from build123d import *

# Parameters (mm, degrees)
BRIDA_BASE1_DEPTH                = 2
REDONDEO5MM_R                    = 5
REDONDEO3MM_R                    = 3
BRIDA_DE_ARISTA1_STRIP_W         = 12
BRIDA_DE_ARISTA1_STRIP_H         = 2
BRIDA_DE_ARISTA1_STRIP_CUT_DEPTH = 30
BRIDA_DE_ARISTA1_DEPTH           = 30
BRIDA_DE_ARISTA2_STRIP_W         = 12
BRIDA_DE_ARISTA2_STRIP_H         = 2
BRIDA_DE_ARISTA2_STRIP_CUT_DEPTH = 18
BRIDA_DE_ARISTA2_DEPTH           = 18
BRIDA_START                      = 2
BRIDA_DE_ARISTA2_FLAT_DEPTH      = 2
CORTAR_EXTRUIR6_REACH            = 43.255
CROQUIS26_R                      = 2
REDONDEO11MM_R                   = 11
TALADRO_ROSCADO_M32_D            = 2.5
TALADRO_ROSCADO_M32_DEPTH        = 20.65
TALADRO_ROSCADO_M32_TIP          = 0.751075774
TALADRO_ROSCADO_M52_D            = 4.2
TALADRO_ROSCADO_M52_DEPTH        = 2
CORTAR_EXTRUIR7_REACH            = 42.274
CROQUIS36_R                      = 2


# Sheet-metal steps are written as plain solids
with BuildPart() as part:
    # Croquis1 → Brida base1 (new body)
    with BuildSketch(Plane.XY):
        with BuildLine():
            Line((0, 0), (30, 0))
            Line((30, 0), (30, 3))
            ThreePointArc((30, 3), (27.886584846, 9.212566007), (24, 14.5))
            Line((24, 14.5), (24, 17))
            Line((24, 17), (6, 17))
            Line((6, 17), (6, 14.5))
            ThreePointArc((6, 14.5), (2.113415154, 9.212566007), (0, 3))
            Line((0, 3), (0, 0))
        make_face()
    extrude(amount=-BRIDA_BASE1_DEPTH)

    # Redondeo5mm
    redondeo5mm_edges = [part.edges().sort_by_distance(p)[0] for p in [
        (0, 3, -1),
        (30, 3, -1),
    ]]
    fillet(redondeo5mm_edges, radius=REDONDEO5MM_R)

    # Redondeo3mm
    redondeo3mm_edges = [part.edges().sort_by_distance(p)[0] for p in [
        (6, 14.5, -1),
        (24, 14.5, -1),
    ]]
    fillet(redondeo3mm_edges, radius=REDONDEO3MM_R)

    # Brida de arista1 strip (across the edge) → Brida de arista1 strip cut (cut)
    with BuildSketch(Plane.YZ):
        with Locations((-4, -1)):
            Rectangle(BRIDA_DE_ARISTA1_STRIP_W, BRIDA_DE_ARISTA1_STRIP_H)
    extrude(amount=BRIDA_DE_ARISTA1_STRIP_CUT_DEPTH, mode=Mode.SUBTRACT)

    # Brida de arista1 section (across the edge) → Brida de arista1 (add)
    with BuildSketch(Plane.YZ):
        with BuildLine():
            Line((-2, 2), (-2, 19))
            Line((-2, 19), (0, 19))
            Line((0, 19), (0, 2))
            ThreePointArc((0, 2), (0.585786438, 0.585786438), (2, 0))
            Line((2, 0), (2, -2))
            ThreePointArc((2, -2), (-0.828427125, -0.828427125), (-2, 2))
        make_face()
    extrude(amount=BRIDA_DE_ARISTA1_DEPTH)

    # Brida de arista2 strip (across the edge) → Brida de arista2 strip cut (cut)
    with BuildSketch(Plane(origin=(24, 17, 0), x_dir=(0, -1, 0), z_dir=(-1, 0, 0))):
        with Locations((-4, -1)):
            Rectangle(BRIDA_DE_ARISTA2_STRIP_W, BRIDA_DE_ARISTA2_STRIP_H)
    extrude(amount=BRIDA_DE_ARISTA2_STRIP_CUT_DEPTH, mode=Mode.SUBTRACT)

    # Brida de arista2 bend section (across the edge) → Brida de arista2 (add)
    with BuildSketch(Plane(origin=(24, 17, 0), x_dir=(0, -1, 0), z_dir=(-1, 0, 0))):
        with BuildLine():
            Line((-2, 2), (0, 2))
            ThreePointArc((0, 2), (0.585786438, 0.585786438), (2, 0))
            Line((2, 0), (2, -2))
            ThreePointArc((2, -2), (-0.828427125, -0.828427125), (-2, 2))
        make_face()
    extrude(amount=BRIDA_DE_ARISTA2_DEPTH)

    # Brida de arista2 profile (on flange) → Brida de arista2 flat (add)
    with BuildSketch(Plane(origin=(0, 17, 0), x_dir=(-1, 0, 0), z_dir=(0, 1, 0)).offset(BRIDA_START)):
        with BuildLine():
            ThreePointArc((-6, 10), (-15, 19), (-24, 10))
            Line((-24, 10), (-24, 2))
            Line((-24, 2), (-6, 2))
            Line((-6, 2), (-6, 10))
        make_face()
    extrude(amount=-BRIDA_DE_ARISTA2_FLAT_DEPTH)

    # Croquis26 → Cortar-Extruir6 (cut, up to next)
    with BuildSketch(Plane(origin=(0, 0, -2), x_dir=(-1, 0, 0), z_dir=(0, 0, -1)), mode=Mode.PRIVATE) as cortar_extruir6_sk1:
        with Locations((-6.25, 8.3)):
            Circle(CROQUIS26_R)
    cortar_extruir6_tool1 = extrude(cortar_extruir6_sk1.sketch, amount=-CORTAR_EXTRUIR6_REACH, mode=Mode.PRIVATE) & part.part
    # Croquis26 → Cortar-Extruir6 (cut, up to next)
    with BuildSketch(Plane(origin=(0, 0, -2), x_dir=(-1, 0, 0), z_dir=(0, 0, -1)), mode=Mode.PRIVATE) as cortar_extruir6_sk2:
        with Locations((-23.75, 8.3)):
            Circle(CROQUIS26_R)
    cortar_extruir6_tool2 = extrude(cortar_extruir6_sk2.sketch, amount=-CORTAR_EXTRUIR6_REACH, mode=Mode.PRIVATE) & part.part
    add(cortar_extruir6_tool1.solids().sort_by_distance((6.25, 8.3, -2))[0], mode=Mode.SUBTRACT)
    add(cortar_extruir6_tool2.solids().sort_by_distance((23.75, 8.3, -2))[0], mode=Mode.SUBTRACT)

    # Redondeo11mm
    redondeo11mm_edges = [part.edges().sort_by_distance(p)[0] for p in [
        (0, -1, 19),
        (30, -1, 19),
    ]]
    fillet(redondeo11mm_edges, radius=REDONDEO11MM_R)

    # Taladro roscado M32
    with Locations(Plane(origin=(0, 0, 0), x_dir=(1, 0, 0), z_dir=(0, 1, 0))):
        with Locations((3.25, -9), (26.75, -9)):
            Hole(TALADRO_ROSCADO_M32_D / 2, depth=TALADRO_ROSCADO_M32_DEPTH)
            with Locations((0, 0, -(TALADRO_ROSCADO_M32_DEPTH + TALADRO_ROSCADO_M32_TIP / 2))):  # 118° drill point
                Cone(0, TALADRO_ROSCADO_M32_D / 2, TALADRO_ROSCADO_M32_TIP, mode=Mode.SUBTRACT)

    # Taladro roscado M52
    with Locations(Plane(origin=(3.715500562, 0, 2.638137214), x_dir=(1, 0, 0), z_dir=(0, 1, 0))):
        with Locations((11.284499438, -7.361862786)):
            Hole(TALADRO_ROSCADO_M52_D / 2, depth=TALADRO_ROSCADO_M52_DEPTH)

    # Croquis36 → Cortar-Extruir7 (cut, up to next)
    with BuildSketch(Plane(origin=(0, 17, 0), x_dir=(1, 0, 0), z_dir=(0, 1, 0)), mode=Mode.PRIVATE) as cortar_extruir7_sk1:
        with Locations(Location((15, -10, 0), (0, 0, 270))):
            Circle(CROQUIS36_R)
    cortar_extruir7_tool1 = extrude(cortar_extruir7_sk1.sketch, amount=CORTAR_EXTRUIR7_REACH, mode=Mode.PRIVATE) & part.part
    add(cortar_extruir7_tool1.solids().sort_by_distance((15, 17, 10))[0], mode=Mode.SUBTRACT)


solid = part.part
For this review, take the finished solid that the model builds, in its own axes (mm). A direction names the side the tool comes from. Give positions to 0.01 mm unless a question says otherwise; leave off trailing zeros. Loops run counter-clockwise (first coordinate to the right, second up) from the corner with the lowest first, then second, coordinate; pieces in that order, holes last. Notation, with made-up numbers: (7.5, 68) - (52.5, 68) arc R9 cw to (52.5, 84) - close; hole circle Ø7 at (19, -9.75). An arc over 180 degrees is marked (long way). Write each question's results on one line, items separated by ' | '.
(1) For pin 1 Ø11 at (x, y) = (21, 10.5) entering from +Z; pin 2 Ø2 at (y, z) = (16.5, 1) entering from -X; pin 3 Ø5 at (x, y) = (8, 11) entering from +Z, all flat-tipped, find the tip position at first contact; note any pin that passes through.
Conclusion:
pin 1: z = 0.27 | pin 2: x = 6 | pin 3: z = 0
(2) Take a section at C-C (z = 11). Give the boundary of the cut face in (x, y), then the cut area to 3 significant figures.
Conclusion:
outline: (0.42, -2) - (13.15, -2) - (13.15, 0) - (0.42, 0) - close; (6.06, 17) - (13.27, 17) - (13.27, 19) - (6.06, 19) - close; (16.73, 17) - (23.94, 17) - (23.94, 19) - (16.73, 19) - close; (16.85, -2) - (29.58, -2) - (29.58, 0) - (16.85, 0) - close | area: 79.8 mm^2
(3) For faces 4 (the cylindrical face through (15.273, -1.014, 7.918)), 5 (the flat face through (24, 18, 4)), 6 (the flat face through (6, 18, 4)), 7 (the cylindrical face through (15, 18, 19)), 8 (the cylindrical face through (14.79, 0.57, 0.6)), list the 3-axis set-ups (+Z, -Z, +X, -X, +Y, -Y) from which the entire face can be reached by the end or side of a thin tool; tool diameter is ignored.
Conclusion:
face 4: -Y | face 5: +Z, -Z, +X, +Y | face 6: +Z, -Z, -X, +Y | face 7: +Z, +Y | face 8: +Z, +X, -X
(4) Take a section at B-B (x = 2.5). Give the boundary of the cut face in (y, z), then the cut area to 3 significant figures.
Conclusion:
outline: (-2, 2) arc R4 ccw to (2, -2) - (9.92, -2) - (9.92, 0) - (2, 0) arc R2 cw to (0, 2) - (0, 8) - (-2, 8) - close; (-2, 10) - (0, 10) - (0, 14.98) - (-2, 14.98) - close | area: 47.2 mm^2
(5) Draft analysis for pull direction X (two halves, no side actions). For faces 1 (the cylindrical face through (15.13, 16.43, 0.6)), 2 (the cylindrical face through (26.863, -0.986, 15.692)), 3 (the cylindrical face through (25.337, 7.083, -1.014)), state which applies: +X half, -X half, draft (parallel to the pull), parting line (faces both ways), or undercut.
Conclusion:
face 1: draft | face 2: +X half | face 3: undercut
(6) Take a section at D-D (z = -0.5). Give the boundary of the cut face in (x, y), then the cut area to 3 significant figures.
Conclusion:
outline: (0, -1.12) - (30, -1.12) - (30, 2.53) arc R5 ccw to (29.9, 3.52) arc R21.53 ccw to (24.77, 13.69) arc R3 cw to (24, 15.7) - (24, 18.12) - (6, 18.12) - (6, 15.7) arc R3 cw to (5.23, 13.69) arc R21.53 ccw to (0.1, 3.52) arc R5 ccw to (0, 2.53) - close; hole circle Ø4 at (6.25, 8.3); hole circle Ø4 at (23.75, 8.3) | area: 457 mm^2
(7) For line 1 along X through (y, z) = (18.55, 10); line 2 along Y through (x, z) = (11, 2.75); line 3 along X through (y, z) = (-0.75, 9), list the stretches that pass through material, from the lowest coordinate up.
Conclusion:
line 1: 6 to 13, 17 to 24 | line 2: -2 to 0, 17 to 19 | line 3: 0.05 to 2, 4.5 to 13.15, 16.85 to 25.5, 28 to 29.95
(8) Take a section at A-A (z = 5.75). Give the boundary of the cut face in (x, y).
Conclusion:
outline: (0, -2) - (30, -2) - (30, 0) - (0, 0) - close; (6, 17) - (24, 17) - (24, 19) - (6, 19) - close
